```python
from build123d import *

# Parameters (mm, degrees)
BOSS_EXTRUDE1_DEPTH            = 10
FILLET1_R                      = 2.5
CUT_EXTRUDE1_DEPTH             = 2.7
CBORE_FOR_M3_SHCS1_D           = 3.4
CBORE_FOR_M3_SHCS1_DEPTH       = 7.6
CBORE_FOR_M3_SHCS1_CBORE_D     = 6.5
CBORE_FOR_M3_SHCS1_CBORE_DEPTH = 3
M3_CLEARANCE_HOLE1_D           = 3.4
M3_CLEARANCE_HOLE1_DEPTH       = 2.3


with BuildPart() as part:
    # Sketch1 → Boss-Extrude1 (new body)
    with BuildSketch(Plane(origin=(0, 0, 0), x_dir=(1, 0, 0), z_dir=(0, 1, 0))):
        with BuildLine():
            Line((5.1, 0), (17, 0))
            Line((17, 0), (17, 7.6))
            Line((17, 7.6), (-23, 7.6))
            Line((-23, 7.6), (-23, -16.5))
            Line((-23, -16.5), (17, -16.5))
            Line((17, -16.5), (17, -11.5))
            Line((17, -11.5), (-17, -11.5))
            Line((-17, -11.5), (-17, 0))
            Line((-17, 0), (-5.1, 0))
            ThreePointArc((-5.1, 0), (0, 5.1), (5.1, 0))
        make_face()
    extrude(amount=BOSS_EXTRUDE1_DEPTH)

    # Fillet1
    fillet1_edges = [part.edges().sort_by_distance(p)[0] for p in [
        (-17, 5, 0),
        (-17, 5, 11.5),
        (17, 5, 11.5),
        (17, 5, 16.5),
        (-23, 5, 16.5),
        (-23, 5, -7.6),
        (17, 5, -7.6),
        (17, 5, 0),
    ]]
    fillet(fillet1_edges, radius=FILLET1_R - 0.0001)  # a hair under: the kernel refuses the full size

    # Sketch3 → Cut-Extrude1 (cut)
    with BuildSketch(Plane(origin=(0, 0, 11.5), x_dir=(-1, 0, 0), z_dir=(0, 0, -1))):
        Polygon((3.3, 5), (1.65, 7.857883832), (-1.65, 7.857883832), (-3.3, 5), (-1.65, 2.142116168), (1.65, 2.142116168), align=None)
    extrude(amount=-CUT_EXTRUDE1_DEPTH, mode=Mode.SUBTRACT)

    # CBORE for M3 SHCS1
    with Locations(Plane.XY):
        with Locations((-9.8, 5), (9.8, 5)):
            CounterBoreHole(CBORE_FOR_M3_SHCS1_D / 2, CBORE_FOR_M3_SHCS1_CBORE_D / 2, CBORE_FOR_M3_SHCS1_CBORE_DEPTH, depth=CBORE_FOR_M3_SHCS1_DEPTH)

    # M3 Clearance Hole1
    with Locations(Plane(origin=(0, 0, 14.2), x_dir=(-1, 0, 0), z_dir=(0, 0, -1))):
        with Locations((0, 5)):
            Hole(M3_CLEARANCE_HOLE1_D / 2, depth=M3_CLEARANCE_HOLE1_DEPTH)


solid = part.part
```
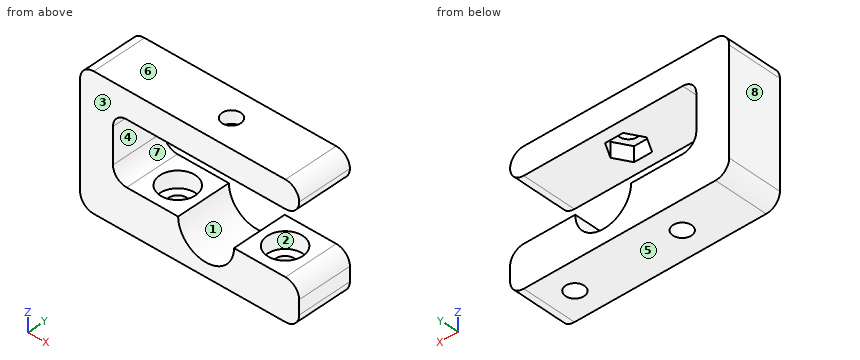
Could you check a few things on this model? Use its own coordinates, in mm. Face numbers are marked on the shaded views. A direction names the side the tool comes from. Round coordinates to 2 decimals unless told otherwise and drop trailing zeros. Order: outer loops, then holes, each group sorted by start corner. A loop starts at its lowest first (then second) coordinate and runs counter-clockwise, first axis right, second up. Notation, with made-up numbers: M 24.5,-9 L 70.5,-9 A19 ccw 70.5,22 Z; hole C 34.25,59 d6. An arc over 180 degrees is marked long. One line per question, with ' | ' between items. Start each with the question number.
(1) For P1, Ø3, axis at x = 0.5, z = 13, coming from the -Y side; P2, Ø5, axis at y = 7, z = 4.5, coming from the +X side; P3, Ø6, axis at y = 5.5, z = 7.5, coming from the +X side; P4, Ø2, axis at x = 0, y = 5, coming from the +Z side, each with a flat end and sliding along its axis, tell me the tip position at first contact or that it passes through.
(2) Please list where these lines run through material, in increasing order: line 1 along Y through (x, z) = (-9.8, -2.3); line 2 along Z through (x, y) = (0, 2.25); line 3 along Y through (x, z) = (9.8, -4.55).
(3) Suppose I cut it at B-B on x = -16. List the corners of the cut face in (y, z) for me, then the cut area to 3 significant figures.
(4) For the marked faces 1, 2, 3 and 4, which set-ups out of +Z, -Z, +X, -X, +Y, -Y let a thin tool reach every point of the face, with its end or its side?
(5) Suppose I cut it at C-C on x = 0. List the corners of the cut face in (y, z) for me, then the cut area to 3 significant figures.
(6) Thinking about a two-plate mould opening in Z: for the marked faces 5, 6, 7 and 8, which applies, +Z half, -Z half, draft (parallel to the pull), parting line (faces both ways), or undercut?
(7) Suppose I cut it at D-D on z = 4. List the corners of the cut face in (x, y) for me.
(8) Suppose I cut it at A-A on x = -9.8. List the corners of the cut face in (y, z) for me.
Geometry results:
1) P1: y = 0 | P2: x = -16.95 | P3: x = -16.5 | P4: z = -5
2) line 1: 0 to 1.75, 8.25 to 10 | line 2: -7.6 to -5.1, 14.2 to 16.5 | line 3: 0 to 3.3, 6.7 to 10
3) outline: M 0,-7.6 L 10,-7.6 L 10,0.5 L 0,0.5 Z; M 0,11 L 10,11 L 10,16.5 L 0,16.5 Z | area: 136 mm²
4) face 1: +Y, -Y | face 2: none | face 3: +Z, -Z, +X, -X, -Y | face 4: +X, +Y, -Y
5) outline: M 0,-7.6 L 10,-7.6 L 10,-5.1 L 0,-5.1 Z; M 0,11.5 L 2.14,11.5 L 2.14,14.2 L 3.3,14.2 L 3.3,16.5 L 0,16.5 Z; M 6.7,14.2 L 7.86,14.2 L 7.86,11.5 L 10,11.5 L 10,16.5 L 6.7,16.5 Z | area: 51.7 mm²
6) face 5: -Z half | face 6: +Z half | face 7: undercut | face 8: draft
7) outline: M -23,0 L -17,0 L -17,10 L -23,10 Z
8) outline: M 0,-7.6 L 3.3,-7.6 L 3.3,-3 L 1.75,-3 L 1.75,0 L 0,0 Z; M 0,11.5 L 10,11.5 L 10,16.5 L 0,16.5 Z; M 6.7,-7.6 L 10,-7.6 L 10,0 L 8.25,0 L 8.25,-3 L 6.7,-3 Z
